```python
from build123d import *

# Parameters (mm, degrees)
SKETCH1_W           = 25.4
SKETCH1_H           = 25.4
BOSS_EXTRUDE1_DEPTH = 482.6
SKETCH2_R           = 6.35
BOSS_EXTRUDE2_DEPTH = 6.35
SKETCH3_W           = 25.4
SKETCH3_H           = 482.6
BOSS_EXTRUDE3_DEPTH = 18.288


with BuildPart() as part:
    # Sketch1 → Boss-Extrude1 (new body)
    with BuildSketch(Plane(origin=(0, 0, 0), x_dir=(1, 0, 0), z_dir=(0, 1, 0))):
        with Locations((12.7, 12.7)):
            Rectangle(SKETCH1_W, SKETCH1_H)
    extrude(amount=BOSS_EXTRUDE1_DEPTH)

    # Sketch2 → Boss-Extrude2 (add)
    with BuildSketch(Plane(origin=(0, 0, -25.4), x_dir=(-1, 0, 0), z_dir=(0, 0, -1))):
        with Locations(Location((-12.7, 469.9, 0), (0, 0, 180))):
            Circle(SKETCH2_R)
    extrude(amount=BOSS_EXTRUDE2_DEPTH)

    # Sketch3 → Boss-Extrude3 (add)
    with BuildSketch(Plane.ZY):
        with Locations((-12.7, 241.3)):
            Rectangle(SKETCH3_W, SKETCH3_H)
    extrude(amount=BOSS_EXTRUDE3_DEPTH)


solid = part.part
```
The model under review builds one solid part; all positions refer to its coordinate system, in mm. Round coordinates to 2 decimals unless told otherwise and drop trailing zeros. Write each loop counter-clockwise with the first axis right and the second up, starting at its lowest first coordinate (ties: lowest second). Pieces come first, ordered by that corner, then holes.
(1) We need section A-A on x = 12.7. Give the boundary of the cut face in (y, z).
(2) We need section C-C on y = 153.5. Give the boundary of the cut face in (x, z), and give its area (3 significant figures).
(3) We need section B-B on y = 469.9. Give the boundary of the cut face in (x, z).
(4) We need section D-D on x = -11.5. Give the boundary of the cut face in (y, z), and give its area (3 significant figures).
(5) Mouldability with a two-part tool opening along X and no side actions: class faces 1 (the cylindrical face through (11.9, 463.6, -28.5)), 2 (the flat face through (-18.288, 245, -13)), 3 (the flat face through (4, 482.6, -13)), 4 (the flat face through (25.4, 238, -13)) as +X half, -X half, draft (parallel to the pull), parting line (faces both ways), or undercut.
(6) Wall thickness on L1, parallel to Z at x = 12, y = 127; L2, parallel to Y at x = 12, z = -26: over which ranges is each line inside the solid? List them lowest first.
(7) Insertion check: pin 1 (22 mm diameter, centred on x = 0, y = 279.5, fed in from -Z); pin 2 (1 mm diameter, centred on x = 14.5, z = -27.5, fed in from +Y). Each pin has a flat end and moves straight along its axis. Give the tip position at first contact, or say it passes through.
Findings below:
1. outline: (0, -25.4) - (463.55, -25.4) - (463.55, -31.75) - (476.25, -31.75) - (476.25, -25.4) - (482.6, -25.4) - (482.6, 0) - (0, 0) - close
2. outline: (-18.29, -25.4) - (25.4, -25.4) - (25.4, 0) - (-18.29, 0) - close
2. area: 1,110 mm2
3. outline: (-18.29, -25.4) - (6.35, -25.4) - (6.35, -31.75) - (19.05, -31.75) - (19.05, -25.4) - (25.4, -25.4) - (25.4, 0) - (-18.29, 0) - close
4. outline: (0, -25.4) - (482.6, -25.4) - (482.6, 0) - (0, 0) - close
4. area: 12,300 mm2
5. face 1: parting line
5. face 2: -X half
5. face 3: draft
5. face 4: +X half
6. L1: z = -25.4 to 0
6. L2: y = 463.59 to 476.21
7. pin 1: stops at z = -25.4
7. pin 2: stops at y = 476.12
